Could you check a few things on this model? Use its own coordinates, in mm. A direction names the side the tool comes from. Give positions to 0.01 mm unless a question says otherwise; leave off trailing zeros. Loops run counter-clockwise (first coordinate to the right, second up) from the corner with the lowest first, then second, coordinate; pieces in that order, holes last. Notation, with made-up numbers: M -6,-27 L 27,-27 A16 ccw 27,-13 Z; hole C -32,-39 d2. An arc over 180 degrees is marked long. Return JSON: item names as keys, results as strings. Group by question number.
1. For pin 1 (1.5 mm diameter, centred on x = 31.5, z = 22, fed in from +Y); pin 2 (12 mm diameter, centred on x = 127.5, z = 27.5, fed in from +Y); pin 3 (8 mm diameter, centred on y = 11.5, z = 27, fed in from +X), each with a flat end and sliding along its axis, tell me the tip position at first contact or that it passes through.
2. For faces 1 (the flat face through (8, 25, 32.5)), 2 (the flat face through (32, 14, 20)), 3 (the flat face through (89, 18, 22)), which set-ups out of +Z, -Z, +X, -X, +Y, -Y let a thin tool reach every point of the face, with its end or its side?
3. If we section it at D-D (x = 127): Write out the boundary of the cut face in (y, z).
4. If we section it at A-A (z = 26.5): Write out the boundary of the cut face in (x, y).
5. If we mould it in two halves opening along Z, with no side actions, what happens to faces 4 (the flat face through (8, 32.5, 25)), 5 (the flat face through (89, 9, 22)), 6 (the flat face through (90, 37, 20))? For each: +Z half, -Z half, draft (parallel to the pull), parting line (faces both ways), or undercut.
6. If we section it at C-C (z = 13): Write out the boundary of the cut face in (x, y) (3 decimals).
7. If we section it at B-B (y = 25): Write out the boundary of the cut face in (x, z).
8. Please list where these lines run through material, in increasing order: line 1 (Y direction, x = 89, z = 29.5); line 2 (X direction, y = 8.5, z = 10.5); line 3 (Z direction, x = 9.5, y = 22).
Solid Edge part; units mm, degrees
sketch "Sketch1" plane through (0, 0, 0) normal (0, -1, 0) x (1, 0, 0)
  line L0 (0, 0) -> (115, 0)
  line L1 (115, 0) -> (115, 50)
  line L2 (115, 50) -> (0, 50)
  line L3 (0, 50) -> (0, 0)
  dimension "D1" = 115
extrude "Protrusion1" add sketch "Sketch1" against normal blind 50
fillet "Verrundung_2" radius 20 4 edges at (57.5, 50, 50) (57.5, 50, 0) (57.5, 0, 50) (57.5, 0, 0)
sketch "Sketch2" plane through (0, 25, 25) normal (-1, 0, 0) x (0, 0, -1)
  line L0 (-7.5, -7.5) -> (7.5, -7.5)
  line L1 (7.5, -7.5) -> (7.5, 7.5)
  line L2 (7.5, 7.5) -> (-7.5, 7.5)
  line L3 (-7.5, 7.5) -> (-7.5, -7.5)
  dimension "D1" = 7.5
extrude "Extrusionsausschnitt_5" cut sketch "Sketch2" against normal blind 15
chamfer "Fase_3" distance 2 angle 45 4 edges at (0, 25, 32.5) (0, 17.5, 25) (0, 25, 17.5) (0, 32.5, 25)
sketch "Sketch3" plane through (115, 25, 25) normal (1, 0, 0) x (0, 1, 0)
  line L0 (-7.5, -7.5) -> (7.5, -7.5)
  line L1 (7.5, -7.5) -> (7.5, 7.5)
  line L2 (7.5, 7.5) -> (-7.5, 7.5)
  line L3 (-7.5, 7.5) -> (-7.5, -7.5)
  dimension "D1" = 7.5
extrude "Extrusionsausprägung_2" add sketch "Sketch3" along normal blind 30
sketch "Sketch4" plane through (57.5, 25, 0) normal (0, 0, -1) x (-1, 0, 0)
  line L0 (-47.5, -17.5) -> (32.5, -17.5)
  line L1 (32.5, -17.5) -> (32.5, 17.5)
  line L2 (32.5, 17.5) -> (-47.5, 17.5)
  line L3 (-47.5, 17.5) -> (-47.5, -17.5)
  dimension "D1" = 32.5
  dimension "D2" = 32.5
extrude "Extrusionsausschnitt_6" cut sketch "Sketch4" against normal blind 20
sketch "Sketch5" plane through (65, 25, 20) normal (0, 0, -1) x (-1, 0, 0)
  circle A0 centre (-24, 11.5) radius 0.9
  circle A1 centre (-24, -11.5) radius 0.9
  circle A2 centre (34, -11.5) radius 0.9
  circle A3 centre (34, 11.5) radius 0.9
  dimension "D1" = 24
extrude "Extrusionsausschnitt_7" cut sketch "Sketch5" against normal blind 15
sketch "Sketch6" plane through (65, 25, 20) normal (0, 0, -1) x (-1, 0, 0)
  line L0 (-40, 17.5) -> (40, 17.5)
  line L1 (40, 17.5) -> (40, -17.5)
  line L2 (40, -17.5) -> (-40, -17.5)
  line L3 (-40, -17.5) -> (-40, 17.5)
  line L4 (-28.5, 7) -> (-19.5, 7)
  line L5 (-19.5, 7) -> (-19.5, 16)
  line L6 (-19.5, 16) -> (-28.5, 16)
  line L7 (-28.5, 16) -> (-28.5, 7)
  line L8 (-28.5, -16) -> (-19.5, -16)
  line L9 (-19.5, -16) -> (-19.5, -7)
  line L10 (-19.5, -7) -> (-28.5, -7)
  line L11 (-28.5, -7) -> (-28.5, -16)
  line L12 (29.5, 7) -> (38.5, 7)
  line L13 (38.5, 7) -> (38.5, 16)
  line L14 (38.5, 16) -> (29.5, 16)
  line L15 (29.5, 16) -> (29.5, 7)
  line L16 (29.5, -16) -> (38.5, -16)
  line L17 (38.5, -16) -> (38.5, -7)
  line L18 (38.5, -7) -> (29.5, -7)
  line L19 (29.5, -7) -> (29.5, -16)
extrude "Extrusionsausschnitt_8" cut sketch "Sketch6" against normal blind 5
sketch "Sketch7" plane through (65, 42.5, 14.6938) normal (0, -1, 0) x (-1, 0, 0)
  line L0 (-40, -10.3062) -> (40, -10.3062)
  line L1 (40, -10.3062) -> (40, 10.3062)
  line L2 (40, 10.3062) -> (-40, 10.3062)
  line L3 (-40, 10.3062) -> (-40, -10.3062)
extrude "Extrusionsausschnitt_9" cut sketch "Sketch7" against normal blind 12
properties material "Nylon, allgemein"
Answer:
{
 "1": {"pin 1": "stops at y = 41", "pin 2": "stops at y = 32.5", "pin 3": "stops at x = 115"},
 "2": {"face 1": "-X", "face 2": "-Z, +Y", "face 3": "-Z"},
 "3": {"outline": "M 17.5,17.5 L 32.5,17.5 L 32.5,32.5 L 17.5,32.5 Z"},
 "4": {"outline": "M 0,0 L 115,0 L 115,17.5 L 145,17.5 L 145,32.5 L 115,32.5 L 115,50 L 0,50 L 0,34.5 L 2,32.5 L 15,32.5 L 15,17.5 L 2,17.5 L 0,15.5 Z; hole C 31,13.5 d1.8; hole C 31,36.5 d1.8; hole C 89,13.5 d1.8; hole C 89,36.5 d1.8"},
 "5": {"face 4": "undercut", "face 5": "draft", "face 6": "-Z half"},
 "6": {"outline": "M 0,1.265 L 115,1.265 L 115,48.735 L 105,48.735 L 105,7.5 L 25,7.5 L 25,48.735 L 0,48.735 Z"},
 "7": {"outline": "M 0,0 L 25,0 L 25,25 L 105,25 L 105,0 L 115,0 L 115,17.5 L 145,17.5 L 145,32.5 L 115,32.5 L 115,50 L 0,50 L 0,34.5 L 2,32.5 L 15,32.5 L 15,17.5 L 2,17.5 L 0,15.5 Z"},
 "8": {"line 1": "y = 0 to 12.6, 14.4 to 35.6, 37.4 to 50", "line 2": "x = 0 to 25, 105 to 115", "line 3": "z = 0 to 17.5, 32.5 to 50"}
}
